Part model, mm, in its own coordinate system. A direction names the side the tool comes from. Coordinates: 2 decimals unless noted, no trailing zeros. Loops run counter-clockwise (first coordinate to the right, second up) from the corner with the lowest first, then second, coordinate; pieces in that order, holes last. Notation, with made-up numbers: (77, 75.25) -> (91, 75.25) arc R27 cw to (91, 98.25) -> close; hole circle Ø1 at (-7, 86). An arc over 180 degrees is marked (long way). One line per question, with ' | ' between items. Start each with the question number.
1) Drop flat-ended pins along their axis: pin 1 (6 mm diameter, centred on x = -10, y = 42, fed in from -Z); pin 2 (8 mm diameter, centred on x = -38.5, y = 30.5, fed in from -Z). Give the stop position or say it passes through.
2) Probe L1, parallel to Y at x = -50.8, z = 22; L2, parallel to X at y = 50.8, z = 26.5; L3, parallel to Z at x = 34.5, y = 35.5. List the from-to ranges inside material, lowest first. Write a range as from..to.
3) 3-axis set-ups, long thin cutter, end or side, ignore diameter. For faces 1 (the face through (27, -43, 7.332)), 2 (the face through (-63.506, -1, 23)): which of +Z, -Z, +X, -X, +Y, -Y reach the whole face in a straight line?
4) Cut at B-B (z = 33). List the corners of the cut face in (x, y).
5) Cut at A-A (x = 53.5). List the corners of the cut face in (y, z).
6) Cut at D-D (x = 0). List the corners of the cut face in (y, z).
7) Cut at C-C (y = 0). List the corners of the cut face in (x, z).
from build123d import *

# Parameters (mm, degrees)
F1_W     = 127
F1_H     = 38.1
F2_DEPTH = 63.5
F5_DEPTH = 50.8
F7_DEPTH = 50.8


with BuildPart() as f2:
    # F1 (on Front) → F2 (new body, symmetric)
    with BuildSketch(Plane.XZ):
        with Locations((-0.005746, 19.05)):
            Rectangle(F1_W, F1_H)
    extrude(amount=F2_DEPTH, both=True)

    # F0 (on Front) → F3 (revolve, cut)
    with BuildSketch(Plane.XZ):
        Polygon((48.160355, 7.332348), (38.1, 1.524), (0, 1.524), (0, 0), (92.567263, 0), (92.567263, 7.332348), align=None)
    revolve(axis=Axis((0, 0, 0.762), (0, 0, -1)), mode=Mode.SUBTRACT)

    # F4 (on Top) → F5 (cut, symmetric)
    with BuildSketch(Plane.XY):
        with BuildLine():
            Line((-50.8, 44.45), (-50.8, 50.8))
            Line((-50.8, 50.8), (-44.45, 50.8))
            ThreePointArc((-44.45, 50.8), (-55.290128, 55.290128), (-50.8, 44.45))
        make_face()
        with BuildLine():
            Line((-44.45, 50.8), (-50.8, 50.8))
            Line((-50.8, 50.8), (-50.8, 44.45))
            ThreePointArc((-50.8, 44.45), (-46.309872, 46.309872), (-44.45, 50.8))
        make_face()
    extrude(amount=F5_DEPTH, both=True, mode=Mode.SUBTRACT)

    # F6 (on Top) → F7 (cut, symmetric)
    with BuildSketch(Plane.XY):
        with BuildLine():
            ThreePointArc((50.8, -44.45), (46.309872, -46.309872), (44.45, -50.8))
            Line((44.45, -50.8), (50.8, -50.8))
            Line((50.8, -50.8), (50.8, -44.45))
        make_face()
        with BuildLine():
            Line((50.8, -50.8), (44.45, -50.8))
            ThreePointArc((44.45, -50.8), (50.8, -57.15), (57.15, -50.8))
            ThreePointArc((57.15, -50.8), (55.290128, -46.309872), (50.8, -44.45))
            Line((50.8, -44.45), (50.8, -50.8))
        make_face()
    extrude(amount=F7_DEPTH, both=True, mode=Mode.SUBTRACT)


solid = f2.part
Reported:
1) pin 1: stops at z = 2.72 | pin 2: stops at z = 5.58
2) L1: y = -63.5..44.45, 57.15..63.5 | L2: x = -63.51..-57.15, -44.45..63.49 | L3: z = 7.33..38.1
3) face 1: -Z | face 2: +Z, -Z, -X, +Y, -Y
4) outline: (-63.51, -63.5) -> (63.49, -63.5) -> (63.49, 63.5) -> (-63.51, 63.5) -> close; hole circle Ø12.7 at (-50.8, 50.8); hole circle Ø12.7 at (50.8, -50.8)
5) outline: (-63.5, 7.33) -> (-56.55, 7.33) -> (-56.55, 38.1) -> (-63.5, 38.1) -> close; (-45.05, 7.33) -> (63.5, 7.33) -> (63.5, 38.1) -> (-45.05, 38.1) -> close
6) outline: (-63.5, 7.33) -> (-48.16, 7.33) -> (-38.1, 1.52) -> (38.1, 1.52) -> (48.16, 7.33) -> (63.5, 7.33) -> (63.5, 38.1) -> (-63.5, 38.1) -> close
7) outline: (-63.51, 7.33) -> (-48.16, 7.33) -> (-38.1, 1.52) -> (38.1, 1.52) -> (48.16, 7.33) -> (63.49, 7.33) -> (63.49, 38.1) -> (-63.51, 38.1) -> close
